Job drawing, mm, ordinate dimensions from the low corner. One solid piece. A direction names the side the tool comes from. Round coordinates to 2 decimals unless told otherwise and drop trailing zeros. Loops run counter-clockwise (first coordinate to the right, second up) from the corner with the lowest first, then second, coordinate; pieces in that order, holes last. Notation, with made-up numbers: (57.25, 22.5) - (109.25, 22.5) arc R25 cw to (109.25, 51.5) - close; hole circle Ø11 at (66, 71). An arc over 180 degrees is marked (long way). One line per question, with ' | ' between items. Start each with the question number.
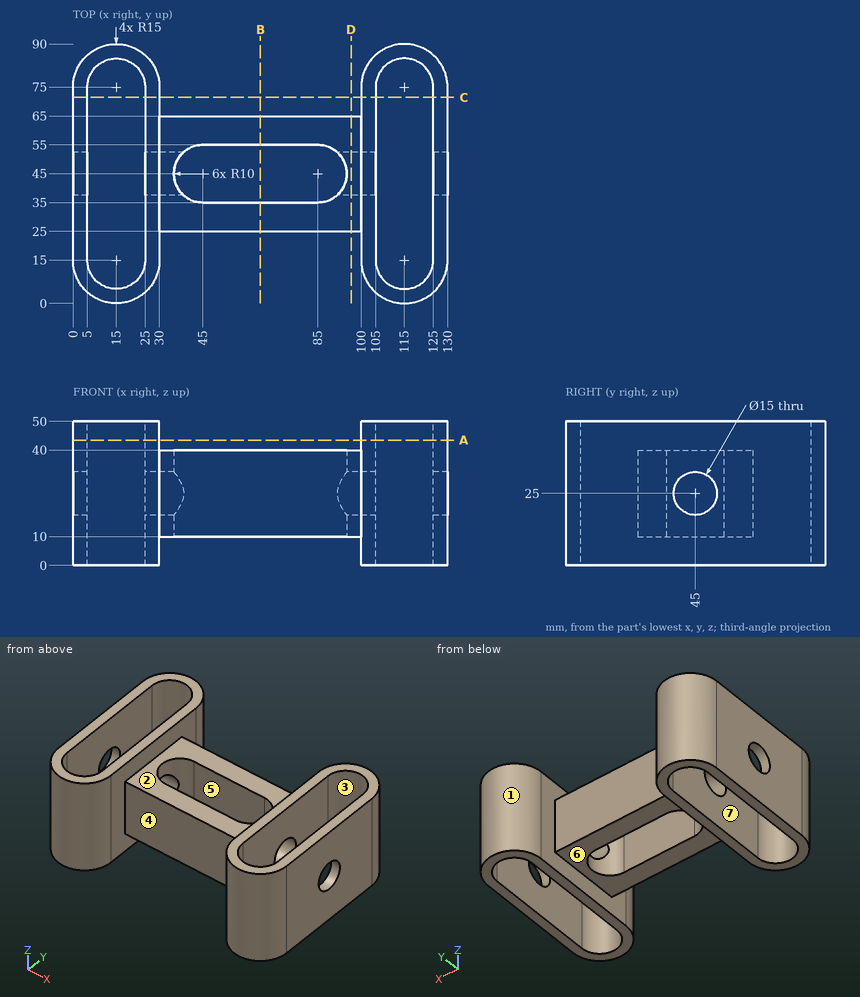
1) Two-plate mould, pull along Y, no slides. Class the marked faces 4, 5, 6 and 7: +Y half, -Y half, draft (parallel to the pull), parting line (faces both ways), or undercut.
2) Wall check: line 1 (X direction, y = 71, z = 31); line 2 (X direction, y = 29, z = 33); line 3 (X direction, y = 53, z = 19.5). Give the ranges that are in metal, low to high. Write a range as [from, to].
3) Drop flat-ended pins along their axis: pin 1 (10 mm diameter, centred on x = 100, z = 16, fed in from +Y); pin 2 (2 mm diameter, centred on x = 39.5, z = 32, fed in from -Y); pin 3 (6 mm diameter, centred on x = 96.5, z = 37, fed in from +Y); pin 4 (10 mm diameter, centred on x = 37.5, y = 73.5, fed in from -Z). Give the stop position or say it passes through.
4) Saw through at C-C on y = 71.5. Write the cut outline in (x, z).
5) Saw through at B-B on x = 65. Write the cut outline in (y, z).
6) Saw through at A-A on z = 43.5. Write the cut outline in (x, y), and give its area (3 significant figures).
7) Saw through at D-D on x = 96.5. Write the cut outline in (y, z).
8) Tool access for the marked faces 1, 2 and 3: list every direction of +Z, -Z, +X, -X, +Y, -Y with a clear straight run to the whole face (end or side of a thin tool).
Answer key:
1) face 4: -Y half | face 5: undercut | face 6: draft | face 7: undercut
2) line 1: [0, 5], [25, 30], [100, 105], [125, 130] | line 2: [0, 5], [25, 105], [125, 130] | line 3: [0, 5], [25, 39], [91, 105], [125, 130]
3) pin 1: y = 86.18 | pin 2: y = 25 | pin 3: y = 65 | pin 4: through
4) outline: (0, 0) - (5, 0) - (5, 50) - (0, 50) - close; (25, 0) - (30, 0) - (30, 50) - (25, 50) - close; (100, 0) - (105, 0) - (105, 50) - (100, 50) - close; (125, 0) - (130, 0) - (130, 50) - (125, 50) - close
5) outline: (25, 10) - (35, 10) - (35, 40) - (25, 40) - close; (55, 10) - (65, 10) - (65, 40) - (55, 40) - close
6) outline: (0, 15) arc R15 ccw to (30, 15) - (30, 75) arc R15 ccw to (0, 75) - close; (100, 15) arc R15 ccw to (130, 15) - (130, 75) arc R15 ccw to (100, 75) - close; hole (5, 15) arc R10 ccw to (25, 15) - (25, 75) arc R10 ccw to (5, 75) - close; hole (105, 15) arc R10 ccw to (125, 15) - (125, 75) arc R10 ccw to (105, 75) - close | area: 1,990 mm²
7) outline: (25, 10) - (65, 10) - (65, 40) - (25, 40) - close; hole circle Ø15 at (45, 25)
8) face 1: +Z, -Z, +Y | face 2: +Z, +Y, -Y | face 3: +Z, -Z
